Design review of the part built by this model. Coordinates are the model's own, in mm. A direction names the side the tool comes from. Coordinates: 2 decimals unless noted, no trailing zeros. Loops run counter-clockwise (first coordinate to the right, second up) from the corner with the lowest first, then second, coordinate; pieces in that order, holes last. Notation, with made-up numbers: (73, -35.75) -> (131, -35.75) arc R22 cw to (131, -15.75) -> close; hole circle Ø1 at (37, -3.75). An arc over 180 degrees is marked (long way). One line per item, written item: value. Start each with the question number.
1. Draft analysis for pull direction X (two halves, no side actions). For faces 4 (the flat face through (3, -7.5, 0)), 5 (the flat face through (5.78, 6.84, 0.42)), 6 (the flat face through (-2.347, 0, 0)), state which applies: pulls with the +X half, pulls with the -X half, needs draft (parallel to the pull), parting line crosses it, or undercut.
2. For probe 1 along Y at (x, z) = (-2.5, 18); probe 2 along X at (y, z) = (-4, -3), list the stretches that pass through material, from the lowest coordinate up.
3. Insertion check: pin 1 (0.6 mm diameter, centred on x = 4.5, z = 6, fed in from +Y); pin 2 (3 mm diameter, centred on x = -5.5, y = 1.5, fed in from -Z). Each pin has a flat end and moves straight along its axis. Give the tip position at first contact, or say it passes through.
4. Add section A-A on x = 0. Write out the cut boundary in (y, z).
5. Machinability: for faces 1 (the flat face through (5, 2.9, 0)), 2 (the flat face through (7.5, -3, 0)), 3 (the flat face through (5.78, -6.84, 0.42)), which of the approach directions +Z, -Z, +X, -X, +Y, -Y give a long, thin tool a straight path to every point of the face, cutting with its end or side? Answer none if there is none.
```python
from build123d import *

# Parameters (mm, degrees)
SKETCH1_W           = 15
SKETCH1_H           = 15
SKETCH1_R           = 1.25
BOSS_EXTRUDE1_DEPTH = 30
FILLET1_R           = 0.25
CUT_EXTRUDE1_DEPTH  = 61
CUT_EXTRUDE3_DEPTH  = 61
FILLET3_R           = 0.5
FILLET4_R           = 0.5
FILLET5_R           = 3
FILLET6_R           = 0.2
CUT_EXTRUDE4_DEPTH  = 61
FILLET8_R           = 0.5
SKETCH6_W           = 5.1529354
SKETCH6_H           = 1.651
SKETCH6_W_2         = 1.651
SKETCH6_H_2         = 5.1529354
CUT_EXTRUDE5_DEPTH  = 61
FILLET10_R          = 0.2


with BuildPart() as part:
    # Sketch1 → Boss-Extrude1 (new body, symmetric)
    with BuildSketch(Plane.XY):
        Rectangle(SKETCH1_W, SKETCH1_H)
        Circle(SKETCH1_R, mode=Mode.SUBTRACT)
    extrude(amount=BOSS_EXTRUDE1_DEPTH, both=True)

    # Fillet1
    fillet1_edges = [part.edges().sort_by_distance(p)[0] for p in [
        (7.5, -7.5, 0),
        (-7.5, -7.5, 0),
        (-7.5, 7.5, 0),
        (7.5, 7.5, 0),
    ]]
    fillet(fillet1_edges, radius=FILLET1_R)

    # Sketch2 → Cut-Extrude1 (cut, through all)
    with BuildSketch(Plane.XY.offset(30)):
        Polygon((-7.5, 1.6), (-6.1, 1.6), (-6.1, 2.9), (-3.4, 2.9), (-3.4, -2.9), (-6.1, -2.9), (-6.1, -1.6), (-7.5, -1.6), align=None)
        Polygon((2.9, 6.1), (1.6, 6.1), (1.6, 7.5), (-1.6, 7.5), (-1.6, 6.1), (-2.9, 6.1), (-2.9, 3.4), (2.9, 3.4), align=None)
        Polygon((-1.6, -7.5), (-1.6, -6.1), (-2.9, -6.1), (-2.9, -3.4), (2.9, -3.4), (2.9, -6.1), (1.6, -6.1), (1.6, -7.5), align=None)
        Polygon((6.1, -2.9), (6.1, -1.6), (7.5, -1.6), (7.5, 1.6), (6.1, 1.6), (6.1, 2.9), (3.4, 2.9), (3.4, -2.9), align=None)
    extrude(amount=-CUT_EXTRUDE1_DEPTH, mode=Mode.SUBTRACT)

    # Sketch4 → Cut-Extrude3 (cut, through all)
    with BuildSketch(Plane.XY.offset(30)):
        Polygon((-3.4, 2.9), (-2.75, 0), (-3.4, -2.9), align=None)
        Polygon((-2.9, 3.4), (0, 2.75), (2.9, 3.4), align=None)
        Polygon((3.4, 2.9), (2.75, 0), (3.4, -2.9), align=None)
        Polygon((-2.9, -3.4), (0, -2.75), (2.9, -3.4), align=None)
    extrude(amount=-CUT_EXTRUDE3_DEPTH, mode=Mode.SUBTRACT)

    # Fillet3
    fillet3_edges = [part.edges().sort_by_distance(p)[0] for p in [
        (1.6, -7.5, 0),
        (-1.6, -7.5, 0),
        (-1.6, -6.1, 0),
        (1.6, -6.1, 0),
        (6.1, 1.6, 0),
        (7.5, 1.6, 0),
        (7.5, -1.6, 0),
        (6.1, -1.6, 0),
        (-7.5, -1.6, 0),
        (-7.5, 1.6, 0),
        (-6.1, 1.6, 0),
        (-6.1, -1.6, 0),
        (-1.6, 6.1, 0),
        (-1.6, 7.5, 0),
        (1.6, 7.5, 0),
        (1.6, 6.1, 0),
    ]]
    fillet(fillet3_edges, radius=FILLET3_R)

    # Fillet4
    fillet4_edges = [part.edges().sort_by_distance(p)[0] for p in [
        (-2.9, -3.4, 0),
        (2.9, -3.4, 0),
        (3.4, -2.9, 0),
        (3.4, 2.9, 0),
        (-3.4, 2.9, 0),
        (-3.4, -2.9, 0),
        (2.9, 3.4, 0),
        (-2.9, 3.4, 0),
    ]]
    fillet(fillet4_edges, radius=FILLET4_R)

    # Fillet5
    fillet5_edges = [part.edges().sort_by_distance(p)[0] for p in [
        (-2.75, 0, 0),
        (0, 2.75, 0),
        (2.75, 0, 0),
        (0, -2.75, 0),
    ]]
    fillet(fillet5_edges, radius=FILLET5_R)

    # Fillet6
    fillet6_edges = [part.edges().sort_by_distance(p)[0] for p in [
        (-2.9, -6.1, 0),
        (2.9, -6.1, 0),
        (6.1, -2.9, 0),
        (6.1, 2.9, 0),
        (-6.1, 2.9, 0),
        (-6.1, -2.9, 0),
        (2.9, 6.1, 0),
        (-2.9, 6.1, 0),
    ]]
    fillet(fillet6_edges, radius=FILLET6_R)

    # Sketch5 → Cut-Extrude4 (cut, through all)
    with BuildSketch(Plane.XY.offset(30)):
        Polygon((-7.5, 6.439339828), (-5.460660172, 4.4), (-7.5, 4.4), align=None)
        Polygon((-6.439339828, 7.5), (-4.4, 5.460660172), (-4.4, 7.5), align=None)
        Polygon((4.4, 7.5), (6.439339828, 7.5), (4.4, 5.460660172), align=None)
        Polygon((7.5, 6.439339828), (7.5, 4.4), (5.460660172, 4.4), align=None)
        Polygon((7.5, -6.439339828), (5.460660172, -4.4), (7.5, -4.4), align=None)
        Polygon((6.439339828, -7.5), (4.4, -5.460660172), (4.4, -7.5), align=None)
        Polygon((-4.4, -7.5), (-6.439339828, -7.5), (-4.4, -5.460660172), align=None)
        Polygon((-7.5, -6.439339828), (-7.5, -4.4), (-5.460660172, -4.4), align=None)
    extrude(amount=-CUT_EXTRUDE4_DEPTH, mode=Mode.SUBTRACT)

    # Fillet8
    fillet8_edges = [part.edges().sort_by_distance(p)[0] for p in [
        (-7.5, 4.4, 0),
        (-7.5, 6.439339828, 0),
        (-5.460660172, 4.4, 0),
        (7.5, -4.4, 0),
        (7.5, -6.439339828, 0),
        (5.460660172, -4.4, 0),
        (5.460660172, 4.4, 0),
        (7.5, 6.439339828, 0),
        (7.5, 4.4, 0),
        (-4.4, 7.5, 0),
        (-4.4, 5.460660172, 0),
        (-6.439339828, 7.5, 0),
        (-5.460660172, -4.4, 0),
        (-7.5, -6.439339828, 0),
        (-7.5, -4.4, 0),
        (4.4, 5.460660172, 0),
        (4.4, 7.5, 0),
        (6.439339828, 7.5, 0),
        (6.439339828, -7.5, 0),
        (4.4, -7.5, 0),
        (4.4, -5.460660172, 0),
        (-6.439339828, -7.5, 0),
        (-4.4, -5.460660172, 0),
        (-4.4, -7.5, 0),
    ]]
    fillet(fillet8_edges, radius=FILLET8_R)

    # Sketch6 → Cut-Extrude5 (cut, through all)
    with BuildSketch(Plane.XY.offset(30)):
        with Locations((4.9235323, 0)):
            Rectangle(SKETCH6_W, SKETCH6_H)
        with Locations((0, -4.9235323)):
            Rectangle(SKETCH6_W_2, SKETCH6_H_2)
        with Locations((-4.9235323, 0)):
            Rectangle(SKETCH6_W, SKETCH6_H)
        with Locations((0, 4.9235323)):
            Rectangle(SKETCH6_W_2, SKETCH6_H_2)
    extrude(amount=-CUT_EXTRUDE5_DEPTH, mode=Mode.SUBTRACT)

    # Fillet10
    fillet10_edges = [part.edges().sort_by_distance(p)[0] for p in [
        (0.8255, -2.935025862, 0),
        (-0.8255, -2.935025862, 0),
        (0.8255, -2.3470646, 0),
        (-0.8255, -2.3470646, 0),
        (2.935025862, 0.8255, 0),
        (2.935025862, -0.8255, 0),
        (2.3470646, 0.8255, 0),
        (2.3470646, -0.8255, 0),
        (-2.935025862, -0.8255, 0),
        (-2.935025862, 0.8255, 0),
        (-2.3470646, -0.8255, 0),
        (-2.3470646, 0.8255, 0),
        (-0.8255, 2.935025862, 0),
        (0.8255, 2.935025862, 0),
        (-0.8255, 2.3470646, 0),
        (0.8255, 2.3470646, 0),
    ]]
    fillet(fillet10_edges, radius=FILLET10_R)


solid = part.part
```
Worked answers:
1. face 4: needs draft
1. face 5: undercut
1. face 6: pulls with the -X half
2. probe 1: y = -7.5 to -6.1, -3.31 to -0.82, 0.82 to 3.31, 6.1 to 7.5
2. probe 2: x = -7.49 to -2.9, 2.9 to 7.49
3. pin 1: stops at y = 7.4
3. pin 2: stops at z = -30
4. outline: (-2.35, -30) -> (-1.25, -30) -> (-1.25, 30) -> (-2.35, 30) -> close; (1.25, -30) -> (2.35, -30) -> (2.35, 30) -> (1.25, 30) -> close
5. face 1: +Z, -Z
5. face 2: +Z, -Z, +X, +Y, -Y
5. face 3: +Z, -Z, -Y
